```python
from build123d import *

# Parameters (mm, degrees)
F0_R     = 5.715
F0_R_2   = 3.175
F1_DEPTH = 9.525
F2_R     = 9.525
F2_R_2   = 5.715
F2_R_3   = 3.175
F3_DEPTH = 1.5875
F4_SIZE  = 0.508
F5_SIZE  = 0.254


with BuildPart() as f1:
    # F0 (on Top) → F1 (new body)
    with BuildSketch(Plane.XY):
        Circle(F0_R)
        Circle(F0_R_2, mode=Mode.SUBTRACT)
    extrude(amount=F1_DEPTH)

    # F2 (on face) → F3 (join)
    with BuildSketch(Plane.XY.offset(9.525)):
        Circle(F2_R)
        Circle(F2_R_2, mode=Mode.SUBTRACT)
        Circle(F2_R_2)
        Circle(F2_R_3, mode=Mode.SUBTRACT)
    extrude(amount=F3_DEPTH)

    # F4
    f4_edges = [f1.edges().sort_by_distance(p)[0] for p in [
        (-9.525, 0, 11.1125),
    ]]
    chamfer(f4_edges, length=F4_SIZE)

    # F5
    f5_edges = [f1.edges().sort_by_distance(p)[0] for p in [
        (-3.175, 0, 11.1125),
        (-5.715, 0, 0),
        (-3.175, 0, 0),
    ]]
    chamfer(f5_edges, length=F5_SIZE)


solid = f1.part
```
Source: CAD feature listing. Evaluate the final solid. Frame: model axes, mm. A direction names the side the tool comes from. Give positions to 0.01 mm unless a question says otherwise; leave off trailing zeros. Loops run counter-clockwise (first coordinate to the right, second up) from the corner with the lowest first, then second, coordinate; pieces in that order, holes last. Notation, with made-up numbers: (53, 29.5) - (103, 29.5) arc R35 ccw to (103, 68.5) - close; hole circle Ø10 at (31, 5.5). An arc over 180 degrees is marked (long way). Use CSV: the item, a comma, the result in double quotes. Start each with the question number.
1. Ray query, L1, parallel to Y at x = 0, z = 5.75 (3 decimals); L2, parallel to X at y = -4.75, z = 5.5; L3, parallel to Z at x = -7.5, y = -4.5 (1 decimal). Return the intervals inside material, ascending.
2. Draft query along Y for faces 3 (the cylindrical face through (-0.69, -3.1, 5.48)), 4 (the cylindrical face through (-7.559, -5.796, 10.057)), 5 (the flat face through (-3, -2, 0)). Return one class per face: +Y half, -Y half, draft (parallel to the pull), parting line (faces both ways), or undercut.
3. Reachability of faces 1 (the flat face through (4, 0, 11.112)), 2 (the cylindrical face through (5.45, 1.72, 4.82)) from +Z, -Z, +X, -X, +Y, -Y: full face, straight path, thin tool, end or side. Return the list, or none.
4. Pin query (flat end, axial travel): pin 1 (3 mm diameter, centred on y = -4, z = 9, fed in from +X); pin 2 (5 mm diameter, centred on x = -4.5, z = 5, fed in from +Y); pin 3 (3 mm diameter, centred on y = 1.5, z = 2.5, fed in from -X) (3 decimals). Return the tip coordinate at first contact, or that it passes through.
5. Section C-C (z = 5.5). Output: boundary loops of the cut face in (x, y) (3 decimals), then the cut area to 3 significant figures.
Response:
1,L1,"-5.715 to -3.175, 3.175 to 5.715"
1,L2,"-3.18 to 3.18"
1,L3,"9.5 to 11.1"
2,face 3,"undercut"
2,face 4,"parting line"
2,face 5,"draft"
3,face 1,"+Z, +X, -X, +Y, -Y"
3,face 2,"-Z"
4,pin 1,"x = 9.16"
4,pin 2,"y = 5.35"
4,pin 3,"x = -5.715"
5,outline,"circle Ø11.43 at (0, 0); hole circle Ø6.35 at (0, 0)"
5,area,"70.9 mm²"
